Source: CAD feature listing. Evaluate the final solid. Frame: model axes, mm. Give positions to 0.01 mm unless a question says otherwise; leave off trailing zeros. Order: outer loops, then holes, each group sorted by start corner. A loop starts at its lowest first (then second) coordinate and runs counter-clockwise, first axis right, second up. Notation, with made-up numbers: M 0.25,-29 L 50.25,-29 A27 ccw 50.25,-2 Z; hole C 56,79 d3. An arc over 180 degrees is marked long. Answer in a Markdown table with one row per item. Add a question column.
(1) Section query D-D, the plane z = 83. Return loops of the section in (x, y), plus the area to 3 significant figures.
(2) Section query C-C, the plane x = 0. Return loops of the section in (y, z), plus the area to 3 significant figures.
(3) Section query B-B, the plane y = 0. Return loops of the section in (x, z).
(4) Pin query (flat end, axial travel): P1, Ø8, axis at x = 9.5, z = 37, coming from the +Y side; P2, Ø4, axis at x = 27.5, z = 81, coming from the -Y side; P3, Ø2, axis at x = 11, y = -62, coming from the -Z side; P4, Ø1, axis at x = 9, z = 28, coming from the -Y side. Return the tip coordinate at first contact, or that it passes through.
(5) Section query A-A, the plane z = 63. Return loops of the section in (x, y).
(6) Material intervals for line 1 along Y through (x, z) = (-22, 67); line 2 along Z through (x, y) = (-7, -42); line 3 along Y through (x, z) = (4, 38), sorted ascending.
(7) Mould query, pull axis Z, two halves, no side actions, for faces 1 (the face through (7.6, 34.4, 86.7)), 2 (the face through (30.235, 23.183, 6.314)), 3 (the face through (-1.24, -93.837, 59.174)), 4 (the face through (-33.575, -10.573, 12.012)). Classes: pulls with the +Z half, pulls with the -Z half, needs draft (parallel to the pull), parting line crosses it, or undercut.
from build123d import *

# Parameters (mm, degrees)
F2_R     = 9.525
F3_DEPTH = 152.4


# Not quite as in the source:
# - a fillet or chamfer that OpenCascade refuses, or shapes differently, is made with other operations: its cross-section is extruded or revolved along the edge and cut away or added


with BuildPart() as f1:
    # F0 (on Front) → F1 (revolve)
    with BuildSketch(Plane.XZ):
        with BuildLine():
            Line((-38.1, 0), (0, 0))
            Line((0, 0), (0, 101.6))
            Line((0, 101.6), (-38.1, 101.6))
            Line((-38.1, 101.6), (-38.1, 87.0632982802))
            ThreePointArc((-38.1, 87.0632982802), (-30.48, 79.4432982802), (-38.1, 71.8232982802))
            Line((-38.1, 71.8232982802), (-38.1, 26.8419931632))
            ThreePointArc((-38.1, 26.8419931632), (-30.48, 19.2219931632), (-38.1, 11.6019931632))
            Line((-38.1, 11.6019931632), (-38.1, 0))
        make_face()
    revolve(axis=Axis((0, 0, 50.8), (0, 0, 1)))

    # F2 (on Front) → F3 (join)
    with BuildSketch(Plane.XZ):
        with Locations((0, 49.7302636504)):
            Circle(F2_R)
    extrude(amount=F3_DEPTH)

    # F4: chamfer of 5.08 on 6 edges, made by hand

    # F4_s1 → F4_t2 (revolve, cut)
    with BuildSketch(Plane.XZ):
        Polygon((-38.1, 96.52), (-33.02, 101.6), (-38.1, 101.6), align=None)
    revolve(axis=Axis((0, 0, 101.6), (0, 0, 1)), mode=Mode.SUBTRACT)

    # F4_s3 → F4_t4 (revolve, cut)
    with BuildSketch(Plane.XZ):
        with BuildLine():
            Line((-35.052, 86.4271436394), (-38.1, 91.0830405454))
            Line((-38.1, 91.0830405454), (-38.1, 87.0632982802))
            ThreePointArc((-38.1, 87.0632982802), (-36.4706968515, 86.8870722727), (-35.052, 86.4271436394))
        make_face()
    revolve(axis=Axis((0, 0, 87.0632982802), (0, 0, 1)), mode=Mode.SUBTRACT)

    # F4_s5 → F4_t6 (revolve, cut)
    with BuildSketch(Plane.XZ):
        with BuildLine():
            Line((-38.1, 7.582250898), (-35.052, 12.2381478041))
            ThreePointArc((-35.052, 12.2381478041), (-36.4706968515, 11.7782191708), (-38.1, 11.6019931632))
            Line((-38.1, 11.6019931632), (-38.1, 7.582250898))
        make_face()
    revolve(axis=Axis((0, 0, 11.6019931632), (0, 0, 1)), mode=Mode.SUBTRACT)

    # F4_s7 → F4_t8 (revolve, cut)
    with BuildSketch(Plane.XZ):
        Polygon((-33.02, 0), (-38.1, 5.08), (-38.1, 0), align=None)
    revolve(axis=Axis((0, 0, 0), (0, 0, 1)), mode=Mode.SUBTRACT)


solid = f1.part
Values follow:
| question | item | result |
|---|---|---|
| 1 | outline | C 0,0 d62.72 |
| 1 | area | 3,090 mm² |
| 2 | outline | M -152.4,40.21 L -38.1,40.21 L -38.1,26.84 A7.62 cw -35.05,12.24 L -38.1,7.58 L -38.1,5.08 L -33.02,0 L 33.02,0 L 38.1,5.08 L 38.1,7.58 L 35.05,12.24 A7.62 cw 38.1,26.84 L 38.1,71.82 A7.62 cw 35.05,86.43 L 38.1,91.08 L 38.1,96.52 L 33.02,101.6 L -33.02,101.6 L -38.1,96.52 L -38.1,91.08 L -35.05,86.43 A7.62 cw -38.1,71.82 L -38.1,59.26 L -152.4,59.26 Z |
| 2 | area | 9,480 mm² |
| 3 | outline | M -38.1,5.08 L -33.02,0 L 33.02,0 L 38.1,5.08 L 38.1,7.58 L 35.05,12.24 A7.62 cw 38.1,26.84 L 38.1,71.82 A7.62 cw 35.05,86.43 L 38.1,91.08 L 38.1,96.52 L 33.02,101.6 L -33.02,101.6 L -38.1,96.52 L -38.1,91.08 L -35.05,86.43 A7.62 cw -38.1,71.82 L -38.1,26.84 A7.62 cw -35.05,12.24 L -38.1,7.58 Z |
| 4 | P1 | stops at y = 37.7 |
| 4 | P2 | stops at y = -17.13 |
| 4 | P3 | passes through |
| 4 | P4 | stops at y = -37.14 |
| 5 | outline | C 0,0 d76.2 |
| 6 | line 1 | y = -31.11 to 31.11 |
| 6 | line 2 | z = 43.27 to 56.19 |
| 6 | line 3 | y = -37.89 to 37.89 |
| 7 | face 1 | undercut |
| 7 | face 2 | needs draft |
| 7 | face 3 | parting line crosses it |
| 7 | face 4 | undercut |
